from build123d import *

# Parameters (mm, degrees)
CUT_EXTRUDE_1_DEPTH      = 16
CUT_EXTRUDE_1_DEPTH_BACK = 16


with BuildPart() as part:
    # Sketch 1 → Revolve 1 (revolve)
    with BuildSketch(Plane.XY, mode=Mode.PRIVATE) as revolve_1_sk:
        Polygon((0, 46), (3, 46), (3, 41), (6.9175, 41), (8, 39.9175), (8, 6), (12, 6), (12, 0), (0, 0), align=None)
    revolve(revolve_1_sk.sketch.rotate(Axis((0, 0, 0), (0, 1, 0)), 270), axis=Axis((0, 0, 0), (0, 1, 0)))

    # Sketch 2 → Cut-Extrude 1 (cut, two sides: drawn at the far end of the back side and taken through both)
    with BuildSketch(Plane.XY.offset(-CUT_EXTRUDE_1_DEPTH_BACK)):
        Polygon((-3, 41), (-1.5, 41), (-1.5, 46), (1.5, 46), (1.5, 41), (3, 41), (3, 49), (-3, 49), align=None)
    extrude(amount=CUT_EXTRUDE_1_DEPTH + CUT_EXTRUDE_1_DEPTH_BACK, mode=Mode.SUBTRACT)


solid = part.part
Verification items for the finished model (mm, model axes). A direction names the side the tool comes from. Coordinates: 2 decimals unless noted, no trailing zeros. Order: outer loops, then holes, each group sorted by start corner. A loop starts at its lowest first (then second) coordinate and runs counter-clockwise, first axis right, second up. Notation, with made-up numbers: M 31,56.25 L 55,56.25 A33 ccw 55,94.25 Z; hole C 15.25,31.25 d5. An arc over 180 degrees is marked long. One line per item, written item: value. Start each with the question number.
Item 1: Access from +Z, -Z, +X, -X, +Y, -Y to the whole of each face (thin tool, end or side, straight path). Record for faces 1 (the cylindrical face through (0, 43, 3)), 2 (the cylindrical face through (-7.81, 22.72, -1.73)), 3 (the flat face through (1.5, 44, 0)).
Item 2: Sectioned sample at A-A on x = 0. Record the cut outline in (y, z).
Item 3: Sectioned sample at B-B on z = 0. Record the cut outline in (x, y), then the cut area to 3 significant figures.
Item 4: Depth check by flat-ended pin: P1, Ø1, axis at x = 8, z = -9.5, coming from the +Y side; P2, Ø2, axis at x = 0, z = -3, coming from the -Y side; P3, Ø12, axis at x = 3.5, y = 36, coming from the +Z side; P4, Ø5, axis at x = 8.5, y = 10, coming from the -Z side. Enter the tip coordinate at first touch or a pass-through.
Item 5: Thickness scan on probe 1 along Y at (x, z) = (-7.25, 7.25); probe 2 along Y at (x, z) = (0.5, -3); probe 3 along Z at (x, y) = (-5.25, 8.5). Record the ranges inside material, lowest first.
Item 6: Sectioned sample at C-C on y = 42.5. Record the cut outline in (x, z).
Item 7: Sectioned sample at D-D on y = 21. Record the cut outline in (x, z), then the cut area to 3 significant figures.
Calculated:
1. face 1: +Z, +Y
1. face 2: +Y
1. face 3: +Z, -Z, +X, +Y
2. outline: M 0,-12 L 6,-12 L 6,-8 L 39.92,-8 L 41,-6.92 L 41,-3 L 46,-3 L 46,3 L 41,3 L 41,6.92 L 39.92,8 L 6,8 L 6,12 L 0,12 Z
3. outline: M -12,0 L 12,0 L 12,6 L 8,6 L 8,39.92 L 6.92,41 L 1.5,41 L 1.5,46 L -1.5,46 L -1.5,41 L -6.92,41 L -8,39.92 L -8,6 L -12,6 Z
3. area: 718 mm^2
4. P1: y = 6
4. P2: y = 0
4. P3: z = 8
4. P4: z = -5.29
5. probe 1: 0 to 6
5. probe 2: 0 to 41
5. probe 3: -6.04 to 6.04
6. outline: M -1.5,-2.6 A3 ccw 1.5,-2.6 L 1.5,2.6 A3 ccw -1.5,2.6 Z
7. outline: C 0,0 d16
7. area: 201 mm^2
